from build123d import *
from build123d import SkipClean  # not in build123d's __all__

# Parameters (mm, degrees)
F0_R     = 27.305
F1_DEPTH = 63.5
F3_DEPTH = 86.614
F4_R     = 5.08
F4_R_2   = 2.8448
F5_DEPTH = 6.35
F6_R     = 8.255
F6_R_2   = 6.35
F7_DEPTH = 25.4
F8_DEPTH = 36.5252
F9_DEPTH = 133.35


# Not quite as in the source:
# - after a boolean that leaves OpenCascade's solid faulty, fix() repairs it


with BuildPart() as f1:
    # F0 (on Front) → F1 (new body)
    with BuildSketch(Plane.XZ):
        Circle(F0_R)
    extrude(amount=F1_DEPTH)

    # F2 (on face) → F3 (cut)
    with BuildSketch(Plane(origin=(0, 0, 0), x_dir=(-1, 0, 0), z_dir=(0, 1, 0))):
        with BuildLine():
            ThreePointArc((-17.2053734765, -6.5146962754), (-17.2403976852, -6.0696715093), (-17.344607899, -5.6356047298))
            ThreePointArc((-17.344607899, -5.6356047298), (-22.8599492679, -6.9597210416), (-17.2053734765, -6.5146962754))
        make_face()
        with BuildLine():
            ThreePointArc((-17.2053734765, 6.5146962754), (-22.8599492679, 6.9597210416), (-17.344607899, 5.6356047298))
            ThreePointArc((-17.344607899, 5.6356047298), (-17.2403976852, 6.0696715093), (-17.2053734765, 6.5146962754))
        make_face()
        with BuildLine():
            ThreePointArc((-9.5468886888, 17.0556962754), (-14.9264240488, 18.3472084491), (-10.7195572031, 14.7542047298))
            ThreePointArc((-10.7195572031, 14.7542047298), (-9.8569533288, 15.7641841018), (-9.5468886888, 17.0556962754))
        make_face()
        with BuildLine():
            ThreePointArc((2.8448, 21.082), (-2.0115773711, 23.0935773711), (0, 18.2372))
            ThreePointArc((0, 18.2372), (2.0115773711, 19.0704226289), (2.8448, 21.082))
        make_face()
        with BuildLine():
            ThreePointArc((15.2364886888, 17.0556962754), (11.1001765152, 19.5904316354), (10.7195572031, 14.7542047298))
            ThreePointArc((10.7195572031, 14.7542047298), (13.6832008625, 14.5209609154), (15.2364886888, 17.0556962754))
        make_face()
        with BuildLine():
            ThreePointArc((22.8949734765, 6.5146962754), (19.6051487104, 9.3244720667), (17.344607899, 5.6356047298))
            ThreePointArc((17.344607899, 5.6356047298), (20.4951982427, 3.7049204841), (22.8949734765, 6.5146962754))
        make_face()
        with BuildLine():
            ThreePointArc((22.8949734765, -6.5146962754), (20.4951982427, -3.7049204841), (17.344607899, -5.6356047298))
            ThreePointArc((17.344607899, -5.6356047298), (19.6051487104, -9.3244720667), (22.8949734765, -6.5146962754))
        make_face()
        with BuildLine():
            ThreePointArc((15.2364886888, -17.0556962754), (13.6832008625, -14.5209609154), (10.7195572031, -14.7542047298))
            ThreePointArc((10.7195572031, -14.7542047298), (11.1001765152, -19.5904316354), (15.2364886888, -17.0556962754))
        make_face()
        with BuildLine():
            ThreePointArc((2.8448, -21.082), (2.0115773711, -19.0704226289), (0, -18.2372))
            ThreePointArc((0, -18.2372), (-2.0115773711, -23.0935773711), (2.8448, -21.082))
        make_face()
        with BuildLine():
            ThreePointArc((-9.5468886888, -17.0556962754), (-9.8569533288, -15.7641841018), (-10.7195572031, -14.7542047298))
            ThreePointArc((-10.7195572031, -14.7542047298), (-14.9264240488, -18.3472084491), (-9.5468886888, -17.0556962754))
        make_face()
    extrude(amount=-F3_DEPTH, mode=Mode.SUBTRACT)

    # F4 (on face) → F5 (join)
    with BuildSketch(Plane.XZ.offset(63.5)):
        with Locations((0, 21.082)):
            Circle(F4_R)
        with Locations((0, 21.082)):
            Circle(F4_R_2, mode=Mode.SUBTRACT)
        with Locations((12.3916886888, 17.0556962754)):
            Circle(F4_R)
        with Locations((12.3916886888, 17.0556962754)):
            Circle(F4_R_2, mode=Mode.SUBTRACT)
        with Locations((20.0501734765, 6.5146962754)):
            Circle(F4_R)
        with Locations((20.0501734765, 6.5146962754)):
            Circle(F4_R_2, mode=Mode.SUBTRACT)
        with Locations((20.0501734765, -6.5146962754)):
            Circle(F4_R)
        with Locations((20.0501734765, -6.5146962754)):
            Circle(F4_R_2, mode=Mode.SUBTRACT)
        with Locations((12.3916886888, -17.0556962754)):
            Circle(F4_R)
        with Locations((12.3916886888, -17.0556962754)):
            Circle(F4_R_2, mode=Mode.SUBTRACT)
        with Locations((0, -21.082)):
            Circle(F4_R)
        with Locations((0, -21.082)):
            Circle(F4_R_2, mode=Mode.SUBTRACT)
        with Locations((-12.3916886888, -17.0556962754)):
            Circle(F4_R)
        with Locations((-12.3916886888, -17.0556962754)):
            Circle(F4_R_2, mode=Mode.SUBTRACT)
        with Locations((-20.0501734765, -6.5146962754)):
            Circle(F4_R)
        with Locations((-20.0501734765, -6.5146962754)):
            Circle(F4_R_2, mode=Mode.SUBTRACT)
        with Locations((-20.0501734765, 6.5146962754)):
            Circle(F4_R)
        with Locations((-20.0501734765, 6.5146962754)):
            Circle(F4_R_2, mode=Mode.SUBTRACT)
        with Locations((-12.3916886888, 17.0556962754)):
            Circle(F4_R)
        with Locations((-12.3916886888, 17.0556962754)):
            Circle(F4_R_2, mode=Mode.SUBTRACT)
    with SkipClean():  # cleaning this boolean's faces spoils the solid; the shape is the same uncleaned
        extrude(amount=F5_DEPTH)

    # F6 (on face) → F7 (join)
    with BuildSketch(Plane.XZ.offset(63.5)):
        Circle(F6_R)
        Circle(F6_R_2, mode=Mode.SUBTRACT)
    extrude(amount=F7_DEPTH)

    add(f1.part.fix(), mode=Mode.REPLACE)

    # F2 (on face) → F8 (cut)
    with BuildSketch(Plane(origin=(0, 0, 0), x_dir=(-1, 0, 0), z_dir=(0, 1, 0))):
        with BuildLine():
            ThreePointArc((-7.6164886888, 17.0556962754), (-16.6464230431, 19.2235917098), (-9.5848965521, 13.1924783239))
            ThreePointArc((-9.5848965521, 13.1924783239), (-8.1369543345, 14.8878008411), (-7.6164886888, 17.0556962754))
        make_face()
        with BuildLine():
            ThreePointArc((-9.5468886888, 17.0556962754), (-9.8569533288, 15.7641841018), (-10.7195572031, 14.7542047298))
            ThreePointArc((-10.7195572031, 14.7542047298), (-14.9264240488, 18.3472084491), (-9.5468886888, 17.0556962754))
        make_face(mode=Mode.SUBTRACT)
        with BuildLine():
            ThreePointArc((4.7752, 21.082), (-3.3765763015, 24.4585763015), (0, 16.3068))
            ThreePointArc((0, 16.3068), (3.3765763015, 17.7054236985), (4.7752, 21.082))
        make_face()
        with BuildLine():
            ThreePointArc((2.8448, 21.082), (2.0115773711, 19.0704226289), (0, 18.2372))
            ThreePointArc((0, 18.2372), (-2.0115773711, 23.0935773711), (2.8448, 21.082))
        make_face(mode=Mode.SUBTRACT)
        with BuildLine():
            ThreePointArc((17.1668886888, 17.0556962754), (10.2237932545, 21.3104306297), (9.5848965521, 13.1924783239))
            ThreePointArc((9.5848965521, 13.1924783239), (14.5595841232, 12.8009619211), (17.1668886888, 17.0556962754))
        make_face()
        with BuildLine():
            ThreePointArc((15.2364886888, 17.0556962754), (13.6832008625, 14.5209609154), (10.7195572031, 14.7542047298))
            ThreePointArc((10.7195572031, 14.7542047298), (11.1001765152, 19.5904316354), (15.2364886888, 17.0556962754))
        make_face(mode=Mode.SUBTRACT)
        with BuildLine():
            ThreePointArc((24.8253734765, 6.5146962754), (19.3031676191, 11.2311056394), (15.5086883999, 5.0390783239))
            ThreePointArc((15.5086883999, 5.0390783239), (20.797179334, 1.7982869114), (24.8253734765, 6.5146962754))
        make_face()
        with BuildLine():
            ThreePointArc((22.8949734765, 6.5146962754), (20.4951982427, 3.7049204841), (17.344607899, 5.6356047298))
            ThreePointArc((17.344607899, 5.6356047298), (19.6051487104, 9.3244720667), (22.8949734765, 6.5146962754))
        make_face(mode=Mode.SUBTRACT)
        with BuildLine():
            ThreePointArc((24.8253734765, -6.5146962754), (20.797179334, -1.7982869114), (15.5086883999, -5.0390783239))
            ThreePointArc((15.5086883999, -5.0390783239), (19.3031676191, -11.2311056394), (24.8253734765, -6.5146962754))
        make_face()
        with BuildLine():
            ThreePointArc((22.8949734765, -6.5146962754), (19.6051487104, -9.3244720667), (17.344607899, -5.6356047298))
            ThreePointArc((17.344607899, -5.6356047298), (20.4951982427, -3.7049204841), (22.8949734765, -6.5146962754))
        make_face(mode=Mode.SUBTRACT)
        with BuildLine():
            ThreePointArc((17.1668886888, -17.0556962754), (14.5595841232, -12.8009619211), (9.5848965521, -13.1924783239))
            ThreePointArc((9.5848965521, -13.1924783239), (10.2237932545, -21.3104306297), (17.1668886888, -17.0556962754))
        make_face()
        with BuildLine():
            ThreePointArc((15.2364886888, -17.0556962754), (11.1001765152, -19.5904316354), (10.7195572031, -14.7542047298))
            ThreePointArc((10.7195572031, -14.7542047298), (13.6832008625, -14.5209609154), (15.2364886888, -17.0556962754))
        make_face(mode=Mode.SUBTRACT)
        with BuildLine():
            ThreePointArc((4.7752, -21.082), (3.3765763015, -17.7054236985), (0, -16.3068))
            ThreePointArc((0, -16.3068), (-3.3765763015, -24.4585763015), (4.7752, -21.082))
        make_face()
        with BuildLine():
            ThreePointArc((2.8448, -21.082), (-2.0115773711, -23.0935773711), (0, -18.2372))
            ThreePointArc((0, -18.2372), (2.0115773711, -19.0704226289), (2.8448, -21.082))
        make_face(mode=Mode.SUBTRACT)
        with BuildLine():
            ThreePointArc((-7.6164886888, -17.0556962754), (-8.1369543345, -14.8878008411), (-9.5848965521, -13.1924783239))
            ThreePointArc((-9.5848965521, -13.1924783239), (-16.6464230431, -19.2235917098), (-7.6164886888, -17.0556962754))
        make_face()
        with BuildLine():
            ThreePointArc((-9.5468886888, -17.0556962754), (-14.9264240488, -18.3472084491), (-10.7195572031, -14.7542047298))
            ThreePointArc((-10.7195572031, -14.7542047298), (-9.8569533288, -15.7641841018), (-9.5468886888, -17.0556962754))
        make_face(mode=Mode.SUBTRACT)
        with BuildLine():
            ThreePointArc((-15.2749734765, -6.5146962754), (-15.3337641125, -5.767690418), (-15.5086883999, -5.0390783239))
            ThreePointArc((-15.5086883999, -5.0390783239), (-24.7665828405, -7.2617021329), (-15.2749734765, -6.5146962754))
        make_face()
        with BuildLine():
            ThreePointArc((-17.2053734765, -6.5146962754), (-22.8599492679, -6.9597210416), (-17.344607899, -5.6356047298))
            ThreePointArc((-17.344607899, -5.6356047298), (-17.2403976852, -6.0696715093), (-17.2053734765, -6.5146962754))
        make_face(mode=Mode.SUBTRACT)
        with BuildLine():
            ThreePointArc((-15.2749734765, 6.5146962754), (-24.7665828405, 7.2617021329), (-15.5086883999, 5.0390783239))
            ThreePointArc((-15.5086883999, 5.0390783239), (-15.3337641125, 5.767690418), (-15.2749734765, 6.5146962754))
        make_face()
        with BuildLine():
            ThreePointArc((-17.2053734765, 6.5146962754), (-17.2403976852, 6.0696715093), (-17.344607899, 5.6356047298))
            ThreePointArc((-17.344607899, 5.6356047298), (-22.8599492679, 6.9597210416), (-17.2053734765, 6.5146962754))
        make_face(mode=Mode.SUBTRACT)
    extrude(amount=-F8_DEPTH, mode=Mode.SUBTRACT)

    add(f1.part.fix(), mode=Mode.REPLACE)

    # F9 (cut): a face of the model
    f9_faces = [f1.faces().sort_by_distance(p)[0] for p in [
        (0, -63.5, 0),
    ]]
    extrude(f9_faces, amount=-F9_DEPTH, mode=Mode.SUBTRACT)


solid = f1.part
Work out the finished part from the listing and answer in its coordinate system (mm). A direction names the side the tool comes from. Round coordinates to 2 decimals unless told otherwise and drop trailing zeros. Write each loop counter-clockwise with the first axis right and the second up, starting at its lowest first coordinate (ties: lowest second). Pieces come first, ordered by that corner, then holes.
1) Given pin 1 Ø7.5 at (x, z) = (0, 21.082) entering from -Y; pin 2 Ø10 at (y, z) = (-74, 1) entering from -X; pin 3 Ø3 at (x, z) = (-21, 18) entering from -Y, each flat-ended and moving along its own axis, determine where each tip first touches the part or whether it passes through.
2) A tool of negligible diameter and unlimited length cuts with its end or side. For faces 1 (the flat face through (2.2, -69.85, -23.3)), 2 (the flat face through (22, -69.85, -9)), 3 (the cylindrical face through (-24.65, -18.01, 7.79)), from which of +Z, -Z, +X, -X, +Y, -Y can it reach the whole face along a straight path? Write none if from no direction.
3) A cutting plane is placed at A-A (z = 0). Give the vertices of the cut face in (x, y) (3 decimals).
4) A cutting plane is placed at B-B (y = -53). Give the number of separate pieces and of enclosed holes in the cut face, plus the area to 3 significant figures.
5) The mould has two halves that part along Z. Classify faces 4 (the flat face through (-18, -69.85, -9)), 5 (the flat face through (0, -36.525, 18)): pulls with the +Z half, pulls with the -Z half, needs draft (parallel to the pull), parting line crosses it, or undercut.
6) Straight lines are drawn through the part: line 1 (Z direction, x = 0, y = -49) (3 decimals); line 2 (Z direction, x = 4, y = -5.5); line 3 (X direction, y = -65.5, z = -5.5). For each, find the intervals that lie inside material, in ascending order.
7) A cutting plane is placed at C-C (x = 13). Give the vertices of the cut face in (y, z), plus the area to 3 significant figures.
Completed:
1. pin 1: stops at y = -69.85
1. pin 2: stops at x = -24.34
1. pin 3: stops at y = -63.5
2. face 1: -Z, +X, -X, -Y
2. face 2: +Z, -Z, +X, -Y
2. face 3: +Y
3. outline: (-27.305, -63.5) - (-8.255, -63.5) - (-8.255, -88.9) - (-6.35, -88.9) - (-6.35, 0) - (-27.305, 0) - close; (6.35, -88.9) - (8.255, -88.9) - (8.255, -63.5) - (27.305, -63.5) - (27.305, 0) - (6.35, 0) - close
4. separate pieces: 1
4. enclosed holes: 11
4. area: 1,960 mm2
5. face 4: needs draft
5. face 5: undercut
6. line 1: z = -27.305 to -23.927, -18.237 to -6.35, 6.35 to 18.237, 23.927 to 27.305
6. line 2: z = -27.01 to -23.69, -18.47 to -4.93, 4.93 to 18.47, 23.69 to 27.01
6. line 3: x = -25.03 to -22.71, -17.39 to -15.07, -6.16 to -3.17, 3.17 to 6.16, 15.07 to 17.39, 22.71 to 25.03
7. outline: (-69.85, -22.1) - (-63.5, -22.1) - (-63.5, -24.01) - (0, -24.01) - (0, -21.79) - (-36.53, -21.79) - (-36.53, -19.83) - (-69.85, -19.83) - close; (-69.85, -14.28) - (-36.53, -14.28) - (-36.53, -12.32) - (0, -12.32) - (0, 12.32) - (-36.53, 12.32) - (-36.53, 14.28) - (-69.85, 14.28) - (-69.85, 12.01) - (-63.5, 12.01) - (-63.5, -12.01) - (-69.85, -12.01) - close; (-69.85, 19.83) - (-36.53, 19.83) - (-36.53, 21.79) - (0, 21.79) - (0, 24.01) - (-63.5, 24.01) - (-63.5, 22.1) - (-69.85, 22.1) - close
7. area: 2,120 mm2
